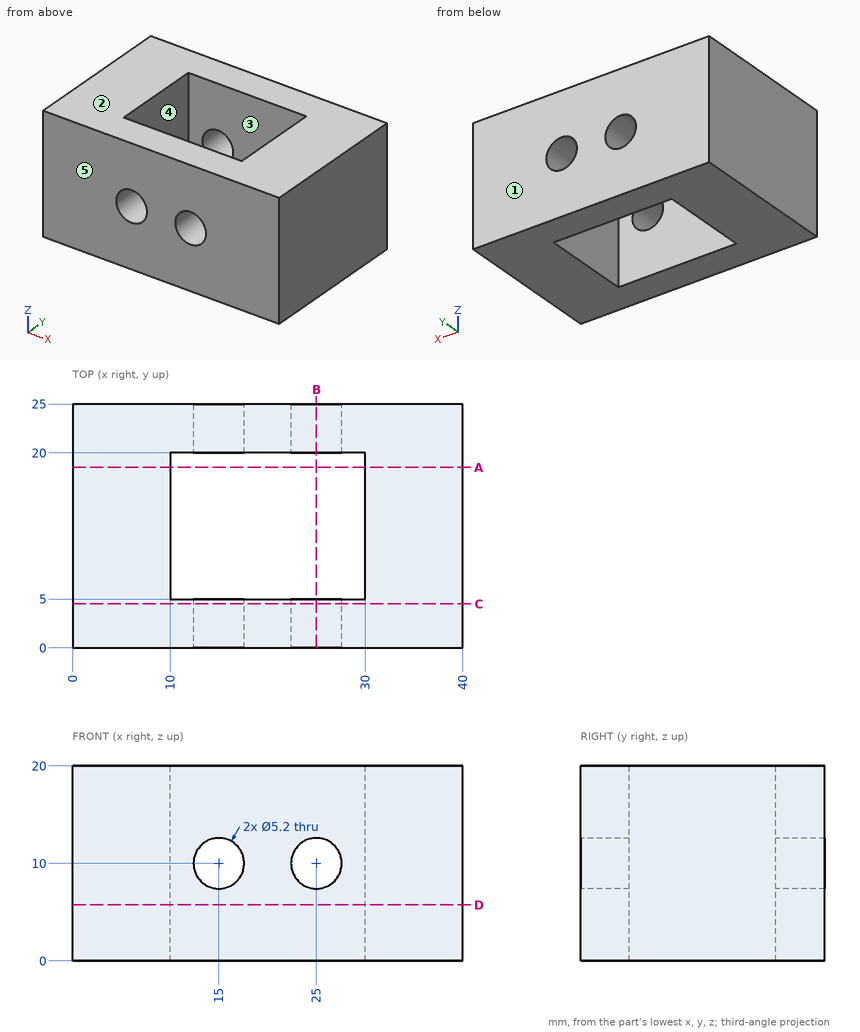
Input: dimensioned drawing with shaded views. Units: mm. Origin: part minimum x, y, z. A direction names the side the tool comes from. Coordinates: 2 decimals unless noted, no trailing zeros. Order: outer loops, then holes, each group sorted by start corner. A loop starts at its lowest first (then second) coordinate and runs counter-clockwise, first axis right, second up. Notation, with made-up numbers: (40, 20.25) - (51, 20.25) arc R31 cw to (51, 48.25) - close; hole circle Ø5 at (72.5, 46). An arc over 180 degrees is marked (long way). Return JSON: item names as keys, results as strings. Group by question number.
1. Cut plane A-A (y = 18.5). Output: boundary loops of the cut face in (x, z), plus the area to 3 significant figures.
2. Set-up query: the marked faces 4 and 5. Return all of +Z, -Z, +X, -X, +Y, -Y with unobstructed straight access to the full face (end or side cutting, diameter ignored); none if empty.
3. Cut plane C-C (y = 4.5). Output: boundary loops of the cut face in (x, z), plus the area to 3 significant figures.
4. Pull-direction query (Y, two-part tool) for the marked faces 1, 2 and 3; classes: pulls with the +Y half, pulls with the -Y half, needs draft (parallel to the pull), parting line crosses it, or undercut.
5. Material intervals for line 1 along Y through (x, z) = (28, 4); line 2 along Z through (x, y) = (25, 23.55); line 3 along X through (y, z) = (15, 11.5), sorted ascending. Write a range as [from, to].
6. Cut plane B-B (x = 25). Output: boundary loops of the cut face in (y, z), plus the area to 3 significant figures.
7. Cut plane D-D (z = 5.75). Output: boundary loops of the cut face in (x, y).
Resolved:
{
 "1": {"outline": "(0, 0) - (10, 0) - (10, 20) - (0, 20) - close; (30, 0) - (40, 0) - (40, 20) - (30, 20) - close", "area": "400 mm²"},
 "2": {"face 4": "+Z, -Z", "face 5": "+Z, -Z, +X, -X, -Y"},
 "3": {"outline": "(0, 0) - (40, 0) - (40, 20) - (0, 20) - close; hole circle Ø5.2 at (15, 10); hole circle Ø5.2 at (25, 10)", "area": "758 mm²"},
 "4": {"face 1": "pulls with the +Y half", "face 2": "needs draft", "face 3": "undercut"},
 "5": {"line 1": "y = [0, 5], [20, 25]", "line 2": "z = [0, 7.4], [12.6, 20]", "line 3": "x = [0, 10], [30, 40]"},
 "6": {"outline": "(0, 0) - (5, 0) - (5, 7.4) - (0, 7.4) - close; (0, 12.6) - (5, 12.6) - (5, 20) - (0, 20) - close; (20, 0) - (25, 0) - (25, 7.4) - (20, 7.4) - close; (20, 12.6) - (25, 12.6) - (25, 20) - (20, 20) - close", "area": "148 mm²"},
 "7": {"outline": "(0, 0) - (40, 0) - (40, 25) - (0, 25) - close; hole (10, 5) - (30, 5) - (30, 20) - (10, 20) - close"}
}
